```python
from build123d import *

# Parameters (mm, degrees)
F1_DEPTH = 63.5
F2_DEPTH = 9.525
F3_DEPTH = 19.05
F0_W     = 31.75
F0_H     = 28.575
F5_R     = 6.35


with BuildPart() as f1:
    # F0 (on Front) → F1 (new body, symmetric)
    with BuildSketch(Plane.XZ):
        Polygon((26.035, 9.525), (-41.275, 9.525), (-41.275, -9.525), (41.275, -9.525), (41.275, 9.525), align=None)
    extrude(amount=F1_DEPTH, both=True)

    # F0 (on Front) → F2 (join, symmetric)
    with BuildSketch(Plane.XZ):
        with BuildLine():
            add(Edge.make_bspline(
                [(-41.275, 9.525), (-16.936806, 41.503267), (15.500731, 69.51972), (50.427763, 74.83017)],
                knots=[0, 0, 0, 0, 111.410759, 111.410759, 111.410759, 111.410759], degree=3))
            Line((-41.275, 9.525), (26.035, 9.525))
            Line((26.035, 9.525), (26.035, 44.45))
            ThreePointArc((26.035, 44.45), (32.887831, 63.930513), (50.427763, 74.83017))
        make_face()
    extrude(amount=F2_DEPTH, both=True)

    # F0 (on Front) → F3 (join, symmetric)
    with BuildSketch(Plane.XZ):
        with BuildLine():
            Line((26.035, 44.45), (26.035, 9.525))
            Line((26.035, 9.525), (41.275, 9.525))
            Line((41.275, 9.525), (41.275, 44.45))
            ThreePointArc((41.275, 44.45), (45.92468, 55.67532), (57.15, 60.325))
            Line((57.15, 60.325), (62.24008, 60.325))
            Line((62.24008, 60.325), (62.24008, 75.565))
            Line((62.24008, 75.565), (57.15, 75.565))
            add(Edge.make_bspline(
                [(50.427763, 74.83017), (52.658838, 75.169392), (54.900071, 75.415964), (57.15, 75.565)],
                knots=[111.410759, 111.410759, 111.410759, 111.410759, 118.527475, 118.527475, 118.527475, 118.527475], degree=3))
            ThreePointArc((50.427763, 74.83017), (32.887831, 63.930513), (26.035, 44.45))
        make_face()
        Polygon((62.24008, 79.375), (62.24008, 75.565), (62.24008, 60.325), (62.24008, 50.8), (93.99008, 50.8), (93.99008, 79.375), align=None)
    extrude(amount=F3_DEPTH, both=True)

    # F0 (on Front) → F4 (revolve)
    with BuildSketch(Plane.XZ):
        with Locations((109.86508, 65.0875)):
            Rectangle(F0_W, F0_H)
    revolve(axis=Axis((93.99008, 0, 65.0875), (0, 0, 1)))

    # F5
    f5_edges = [f1.edges().sort_by_distance(p)[0] for p in [
        (41.275, 63.5, 0),
        (-41.275, 63.5, 0),
        (41.275, -63.5, 0),
        (-41.275, -63.5, 0),
    ]]
    fillet(f5_edges, radius=F5_R)


solid = f1.part
```
Work out the finished part from the listing and answer in its coordinate system (mm). A direction names the side the tool comes from. Give positions to 0.01 mm unless a question says otherwise; leave off trailing zeros. Loops run counter-clockwise (first coordinate to the right, second up) from the corner with the lowest first, then second, coordinate; pieces in that order, holes last. Notation, with made-up numbers: (-27, 44.25) -> (-17, 44.25) arc R30 ccw to (-17, 66.25) -> close; hole circle Ø8 at (37, 89.5). An arc over 180 degrees is marked (long way). Write item = value, one per line. Start each with the question number.
(1) Find section A-A on y = 43. Give the vertices of the cut face in (x, z) (3 decimals), and give its area (3 significant figures).
(2) Find the intervals of material crossed by probe 1 along X at (y, z) = (41, -6) (3 decimals); probe 2 along Y at (x, z) = (23.5, 36) (3 decimals), in increasing order. Write a range as from..to.
(3) Given pin 1 Ø2 at (y, z) = (5, 36) entering from +X (3 decimals); pin 2 Ø16 at (x, y) = (-13.5, -40.5) entering from +Z (3 decimals); pin 3 Ø5 at (y, z) = (16.5, 19.5) entering from -X (3 decimals), each flat-ended and moving along its own axis, determine where each tip first touches the part or whether it passes through.
(4) Which of the six approach directions +Z, -Z, +X, -X, +Y, -Y give full straight-line access (tool end or side, diameter ignored) to faces 1 (the cylindrical face through (45.8, -0.27, 55.55)), 2 (the flat face through (60, 0, 75.565)), 3 (the flat face through (94, 0, 50.8)), 4 (the flat face through (1, 36, 9.525))?
(5) Find section B-B on x = 84. Give the vertices of the cut face in (y, z) (3 decimals).
From the geometry:
q1.outline = (-41.275, -9.525) -> (41.275, -9.525) -> (41.275, 9.525) -> (-41.275, 9.525) -> close
q1.area = 1,570 mm^2
q2.probe_1 = -41.275..41.275
q2.probe_2 = -9.525..9.525
q3.pin_1 = 41.275
q3.pin_2 = 9.525
q3.pin_3 = 26.035
q4.face_1 = -Z, +Y, -Y
q4.face_2 = +Z, -X, +Y, -Y
q4.face_3 = -Z, +X, +Y, -Y
q4.face_4 = +Z, -X, +Y
q5.outline = (-30.137, 50.8) -> (30.137, 50.8) -> (30.137, 79.375) -> (-30.137, 79.375) -> close
